```python
from build123d import *

# Parameters (mm, degrees)
SKETCH2_R            = 39.5
BOSS_EXTRUDE2_DEPTH  = 1
SKETCH6_R            = 41.25
BOSS_EXTRUDE3_DEPTH  = 1
SKETCH7_R            = 42
BOSS_EXTRUDE4_DEPTH  = 7
SKETCH8_R            = 35
BOSS_EXTRUDE5_DEPTH  = 3
BOSS_EXTRUDE6_DEPTH  = 1
CIRPATTERN1_COUNT    = 16
SKETCH10_W           = 20
SKETCH10_H           = 40
BOSS_EXTRUDE7_DEPTH  = 42
SKETCH11_R           = 20
BOSS_EXTRUDE8_DEPTH  = 20
SKETCH12_R           = 10
BOSS_EXTRUDE10_DEPTH = 10
SKETCH13_R           = 10
BOSS_EXTRUDE11_DEPTH = 10
BOSS_EXTRUDE12_START = 10
SKETCH14_R           = 10
BOSS_EXTRUDE12_DEPTH = 10


with BuildPart() as part:
    # Sketch1 → Revolve1 (revolve)
    with BuildSketch(Plane(origin=(0, 0, 0), x_dir=(1, 0, 0), z_dir=(0, 1, 0))):
        with BuildLine():
            Line((0, 0), (0, -20))
            Line((0, -20), (-42, -20))
            ThreePointArc((-42, -20), (-39.360679775, -8.819660113), (-32, 0))
            Line((-32, 0), (0, 0))
        make_face()
    revolve(axis=Axis((0, 0, 0), (0, 0, 1)))

    # Sketch2 → Boss-Extrude2 (add)
    with BuildSketch(Plane.XY.offset(20)):
        Circle(SKETCH2_R)
    extrude(amount=BOSS_EXTRUDE2_DEPTH)

    # Sketch5 → Revolve2 (revolve)
    with BuildSketch(Plane(origin=(0, 0, 0), x_dir=(1, 0, 0), z_dir=(0, 1, 0))):
        with BuildLine():
            Line((0, -20), (-40, -20))
            ThreePointArc((-40, -20), (-41.376973739, -30), (-40, -40))
            Line((-40, -40), (0, -40))
            Line((0, -40), (0, -20))
        make_face()
    revolve(axis=Axis((0, 0, 20), (0, 0, 1)))

    # Sketch6 → Boss-Extrude3 (add)
    with BuildSketch(Plane.XY.offset(40)):
        Circle(SKETCH6_R)
    extrude(amount=BOSS_EXTRUDE3_DEPTH)

    # Sketch7 → Boss-Extrude4 (add)
    with BuildSketch(Plane.XY.offset(41)):
        Circle(SKETCH7_R)
    extrude(amount=BOSS_EXTRUDE4_DEPTH)

    # Sketch8 → Boss-Extrude5 (add)
    with BuildSketch(Plane.XY.offset(48)):
        Circle(SKETCH8_R)
    extrude(amount=BOSS_EXTRUDE5_DEPTH)

    # Sketch9 → Boss-Extrude6 (add)
    with BuildSketch(Plane.XY.offset(48)):
        with BuildLine():
            ThreePointArc((37, 0), (38.5, 1.5), (40, 0))
            Line((40, 0), (40.75, 0))
            ThreePointArc((40.75, 0), (38.5, 2.25), (36.25, 0))
            Line((36.25, 0), (37, 0))
        make_face()
        with BuildLine():
            Line((40.75, 0), (40, 0))
            ThreePointArc((40, 0), (38.5, -1.5), (37, 0))
            Line((37, 0), (36.25, 0))
            ThreePointArc((36.25, 0), (38.5, -2.25), (40.75, 0))
        make_face()
    boss_extrude6 = extrude(amount=BOSS_EXTRUDE6_DEPTH)

    # CirPattern1: Boss-Extrude6 ×16 about axis
    cirpattern1_axis = Axis((0, 0, 0), (0, 0, 1))
    for i in range(1, CIRPATTERN1_COUNT):
        add(boss_extrude6.rotate(cirpattern1_axis, i * 360 / CIRPATTERN1_COUNT))

    # Sketch10 → Boss-Extrude7 (add)
    with BuildSketch(Plane(origin=(0, 0, 0), x_dir=(-1, 0, 0), z_dir=(0, 0, -1))):
        Rectangle(SKETCH10_W, SKETCH10_H)
    extrude(amount=BOSS_EXTRUDE7_DEPTH)

    # Sketch11 → Boss-Extrude8 (add)
    with BuildSketch(Plane.ZY.offset(10)):
        with Locations((-42, 0)):
            Circle(SKETCH11_R)
    extrude(amount=-BOSS_EXTRUDE8_DEPTH)

    # Sketch12 → Boss-Extrude10 (add)
    with BuildSketch(Plane.ZY.offset(10)):
        with Locations(Location((-42, 0, 0), (0, 0, 90))):
            Circle(SKETCH12_R)
    extrude(amount=BOSS_EXTRUDE10_DEPTH)

    # Sketch13 → Boss-Extrude11 (add)
    with BuildSketch(Plane.XY.offset(51)):
        Circle(SKETCH13_R)
    extrude(amount=BOSS_EXTRUDE11_DEPTH)

    # Sketch14 → Boss-Extrude12 (add)
    with BuildSketch(Plane(origin=(10, 0, 0), x_dir=(0, 0, -1), z_dir=(1, 0, 0)).offset(BOSS_EXTRUDE12_START)):
        with Locations(Location((42, 0, 0), (0, 0, 90))):
            Circle(SKETCH14_R)
    extrude(amount=-BOSS_EXTRUDE12_DEPTH)


solid = part.part
```
Check sheet for the modelled part. Datum: model origin and axes. Units: mm. A direction names the side the tool comes from. Give positions to 0.01 mm unless a question says otherwise; leave off trailing zeros. Order: outer loops, then holes, each group sorted by start corner. A loop starts at its lowest first (then second) coordinate and runs counter-clockwise, first axis right, second up. Notation, with made-up numbers: (50.25, 63.5) -> (73.25, 63.5) arc R22 cw to (73.25, 86.5) -> close; hole circle Ø5 at (42.25, 35). An arc over 180 degrees is marked (long way). Use CSV: the item, a comma, the result in double quotes. Start each with the question number.
1) Material ranges on line 1 (Y direction, x = 38.5, z = 48.6); line 2 (X direction, y = -0.5, z = -46); line 3 (X direction, y = -6, z = -28.5), recorded low to high. Write a range as from..to.
2) Set-up check for faces 5 (the face through (-20, 0, -42)), 6 (the face through (-27.32, 29.47, 48.49)), 7 (the face through (0, 20, -21)), 8 (the face through (37, -16, 49)): record each of +Z, -Z, +X, -X, +Y, -Y from which the full face is reachable in a straight line by a thin tool's end or side.
3) Mould release check, pull along Z, two halves, no side actions. Record for faces 1 (the face through (-39, 0, 48)), 2 (the face through (-8.94, -40.27, 40.49)), 3 (the face through (-37.07, 14.73, 48.49)), 4 (the face through (-34, 22, 40)): released by +Z, released by -Z, zero draft, split by the parting line, or undercut.
4) Sectioned sample at A-A, the plane z = -15. Record the boundary of the cut face in (x, y).
5) Go/stop test with flat-tipped pins: P1, Ø3.5, axis at x = -27.22, y = -27.22, coming from the -Z side; P2, Ø1.5, axis at x = -35.5, y = 15, coming from the +Z side; P3, Ø3, axis at x = 19.5, y = -15, coming from the -Z side. Record where each tip stops, or that it passes through.
Recorded:
1,line 1,"-2.25..-1.5, 1.5..2.25"
1,line 2,"-20..20"
1,line 3,"-10..10"
2,face 5,"-Z, -X, +Y, -Y"
2,face 6,"+Z"
2,face 7,"-Z, +X, -X, +Y"
2,face 8,"+Z, +X, -Y"
3,face 1,"released by +Z"
3,face 2,"undercut"
3,face 3,"zero draft"
3,face 4,"undercut"
4,outline,"(-10, -20) -> (10, -20) -> (10, 20) -> (-10, 20) -> close"
5,P1,"z = 4.67"
5,P2,"z = 48"
5,P3,"z = 0"
